Design review of the part built by this model. Coordinates are the model's own, in mm. Face numbers are marked on the shaded views. A direction names the side the tool comes from. Round coordinates to 2 decimals unless told otherwise and drop trailing zeros. Write each loop counter-clockwise with the first axis right and the second up, starting at its lowest first coordinate (ties: lowest second). Pieces come first, ordered by that corner, then holes. Notation, with made-up numbers: (-24, 33) - (-4, 33) arc R27 cw to (-4, 71) - close; hole circle Ø4 at (-13, 87.25). An arc over 180 degrees is marked (long way). Use one line per item in the form item = value.
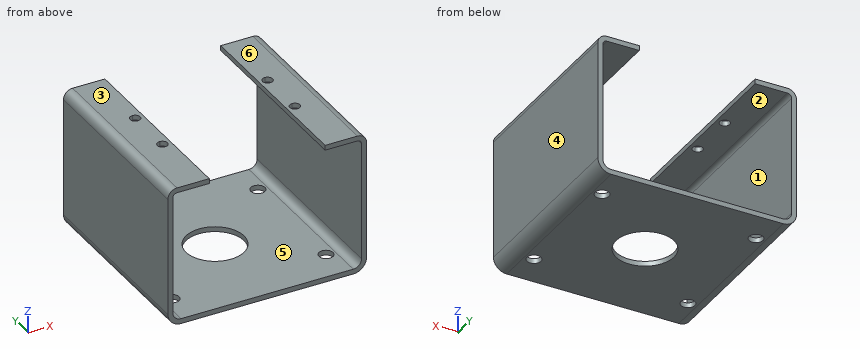
```python
from build123d import *

# Parameters (mm, degrees)
SKETCH1_W                      = 120
SKETCH1_H                      = 115
BASE_FLANGE1_DEPTH             = 3
EDGE_FLANGE1_STRIP_W           = 22
EDGE_FLANGE1_STRIP_H           = 3
EDGE_FLANGE1_STRIP_CUT_DEPTH   = 115
EDGE_FLANGE1_STRIP_2_W         = 22
EDGE_FLANGE1_STRIP_2_H         = 3
EDGE_FLANGE1_STRIP_CUT_2_DEPTH = 115
EDGE_FLANGE1_DEPTH             = 115
EDGE_FLANGE1_BEND_DEPTH        = 115
EDGE_FLANGE2_STRIP_W           = 17
EDGE_FLANGE2_STRIP_H           = 3
EDGE_FLANGE2_STRIP_CUT_DEPTH   = 115
EDGE_FLANGE2_STRIP_2_W         = 17
EDGE_FLANGE2_STRIP_2_H         = 3
EDGE_FLANGE2_STRIP_CUT_2_DEPTH = 115
EDGE_FLANGE2_DEPTH             = 115
EDGE_FLANGE2_BEND_DEPTH        = 115
CUT_EXTRUDE1_DEPTH             = 10
LPATTERN1_COUNT                = 2
LPATTERN1_PITCH                = 30
LPATTERN2_COUNT                = 2
LPATTERN2_PITCH                = 80
LPATTERN2_COPY_1_DEPTH         = 10
SKETCH19_R                     = 4.25
CUT_EXTRUDE2_DEPTH             = 10
LPATTERN3_COUNT                = 2
LPATTERN3_PITCH                = 75
SKETCH20_R                     = 17.5
CUT_EXTRUDE3_DEPTH             = 10


# Sheet-metal steps are written as plain solids
with BuildPart() as part:
    # Sketch1 → Base-Flange1 (new body)
    with BuildSketch(Plane.XY):
        Rectangle(SKETCH1_W, SKETCH1_H)
    extrude(amount=-BASE_FLANGE1_DEPTH)

    # Edge-Flange1 strip (across the edge) → Edge-Flange1 strip cut (cut)
    with BuildSketch(Plane(origin=(60, -57.5, 0), x_dir=(-1, 0, 0), z_dir=(0, 1, 0))):
        with Locations((-3, -1.5)):
            Rectangle(EDGE_FLANGE1_STRIP_W, EDGE_FLANGE1_STRIP_H)
    extrude(amount=EDGE_FLANGE1_STRIP_CUT_DEPTH, mode=Mode.SUBTRACT)

    # Edge-Flange1 strip 2 (across the edge) → Edge-Flange1 strip cut 2 (cut)
    with BuildSketch(Plane(origin=(-60, 57.5, 0), x_dir=(1, 0, 0), z_dir=(0, -1, 0))):
        with Locations((-3, -1.5)):
            Rectangle(EDGE_FLANGE1_STRIP_2_W, EDGE_FLANGE1_STRIP_2_H)
    extrude(amount=EDGE_FLANGE1_STRIP_CUT_2_DEPTH, mode=Mode.SUBTRACT)

    # Edge-Flange1 section (across the edge) → Edge-Flange1 (add)
    with BuildSketch(Plane(origin=(60, -57.5, 0), x_dir=(-1, 0, 0), z_dir=(0, 1, 0))):
        with BuildLine():
            Line((0, 5), (0, 82))
            Line((0, 82), (3, 82))
            Line((3, 82), (3, 5))
            ThreePointArc((3, 5), (4.464466094, 1.464466094), (8, 0))
            Line((8, 0), (8, -3))
            ThreePointArc((8, -3), (2.343145751, -0.656854249), (0, 5))
        make_face()
    extrude(amount=EDGE_FLANGE1_DEPTH)

    # Edge-Flange1 section 2 (across the edge) → Edge-Flange1 bend (add)
    with BuildSketch(Plane(origin=(-60, 57.5, 0), x_dir=(1, 0, 0), z_dir=(0, -1, 0))):
        with BuildLine():
            Line((0, 5), (0, 82))
            Line((0, 82), (3, 82))
            Line((3, 82), (3, 5))
            ThreePointArc((3, 5), (4.464466094, 1.464466094), (8, 0))
            Line((8, 0), (8, -3))
            ThreePointArc((8, -3), (2.343145751, -0.656854249), (0, 5))
        make_face()
    extrude(amount=EDGE_FLANGE1_BEND_DEPTH)

    # Edge-Flange2 strip (across the edge) → Edge-Flange2 strip cut (cut)
    with BuildSketch(Plane(origin=(-57, 57.5, 82), x_dir=(0, 0, -1), z_dir=(0, -1, 0))):
        with Locations((-3, -1.5)):
            Rectangle(EDGE_FLANGE2_STRIP_W, EDGE_FLANGE2_STRIP_H)
    extrude(amount=EDGE_FLANGE2_STRIP_CUT_DEPTH, mode=Mode.SUBTRACT)

    # Edge-Flange2 strip 2 (across the edge) → Edge-Flange2 strip cut 2 (cut)
    with BuildSketch(Plane(origin=(57, -57.5, 82), x_dir=(0, 0, -1), z_dir=(0, 1, 0))):
        with Locations((-3, -1.5)):
            Rectangle(EDGE_FLANGE2_STRIP_2_W, EDGE_FLANGE2_STRIP_2_H)
    extrude(amount=EDGE_FLANGE2_STRIP_CUT_2_DEPTH, mode=Mode.SUBTRACT)

    # Edge-Flange2 section (across the edge) → Edge-Flange2 (add)
    with BuildSketch(Plane(origin=(-57, 57.5, 82), x_dir=(0, 0, -1), z_dir=(0, -1, 0))):
        with BuildLine():
            Line((0, 2.5), (0, 22))
            Line((0, 22), (3, 22))
            Line((3, 22), (3, 2.5))
            ThreePointArc((3, 2.5), (3.732233047, 0.732233047), (5.5, 0))
            Line((5.5, 0), (5.5, -3))
            ThreePointArc((5.5, -3), (1.610912703, -1.389087297), (0, 2.5))
        make_face()
    extrude(amount=EDGE_FLANGE2_DEPTH)

    # Edge-Flange2 section 2 (across the edge) → Edge-Flange2 bend (add)
    with BuildSketch(Plane(origin=(57, -57.5, 82), x_dir=(0, 0, -1), z_dir=(0, 1, 0))):
        with BuildLine():
            Line((0, 2.5), (0, 22))
            Line((0, 22), (3, 22))
            Line((3, 22), (3, 2.5))
            ThreePointArc((3, 2.5), (3.732233047, 0.732233047), (5.5, 0))
            Line((5.5, 0), (5.5, -3))
            ThreePointArc((5.5, -3), (1.610912703, -1.389087297), (0, 2.5))
        make_face()
    extrude(amount=EDGE_FLANGE2_BEND_DEPTH)

    # Sketch18 → Cut-Extrude1 (cut)
    with BuildSketch(Plane.XY.offset(82)):
        with BuildLine():
            Line((-40.05, -12), (-39.95, -12))
            ThreePointArc((-39.95, -12), (-36.95, -15), (-39.95, -18))
            Line((-39.95, -18), (-40.05, -18))
            ThreePointArc((-40.05, -18), (-43.05, -15), (-40.05, -12))
        make_face()
    cut_extrude1 = extrude(amount=-CUT_EXTRUDE1_DEPTH, mode=Mode.SUBTRACT)

    # LPattern1: Cut-Extrude1 ×2
    with Locations(*[(0, i * LPATTERN1_PITCH, 0) for i in range(1, LPATTERN1_COUNT)]):
        add(cut_extrude1, mode=Mode.SUBTRACT)

    # LPattern2: Cut-Extrude1 ×2
    with Locations(*[(i * LPATTERN2_PITCH, 0, 0) for i in range(1, LPATTERN2_COUNT)]):
        add(cut_extrude1, mode=Mode.SUBTRACT)

    # LPattern2 copy 1 sketch → LPattern2 copy 1 (cut)
    with BuildSketch(Plane(origin=(80, 30, 82), x_dir=(1, 0, 0), z_dir=(0, 0, 1))):
        with BuildLine():
            Line((-40.05, -12), (-39.95, -12))
            ThreePointArc((-39.95, -12), (-36.95, -15), (-39.95, -18))
            Line((-39.95, -18), (-40.05, -18))
            ThreePointArc((-40.05, -18), (-43.05, -15), (-40.05, -12))
        make_face()
    extrude(amount=-LPATTERN2_COPY_1_DEPTH, mode=Mode.SUBTRACT)

    # Sketch19 → Cut-Extrude2 (cut)
    with BuildSketch(Plane(origin=(0, 0, -3), x_dir=(-1, 0, 0), z_dir=(0, 0, -1))):
        with Locations((-46.5, -37.5)):
            Circle(SKETCH19_R)
        with Locations((46.5, -37.5)):
            Circle(SKETCH19_R)
    cut_extrude2 = extrude(amount=-CUT_EXTRUDE2_DEPTH, mode=Mode.SUBTRACT)

    # LPattern3: Cut-Extrude2 ×2
    with Locations(*[(0, i * LPATTERN3_PITCH, 0) for i in range(1, LPATTERN3_COUNT)]):
        add(cut_extrude2, mode=Mode.SUBTRACT)

    # Sketch20 → Cut-Extrude3 (cut)
    with BuildSketch(Plane(origin=(0, 0, -3), x_dir=(-1, 0, 0), z_dir=(0, 0, -1))):
        Circle(SKETCH20_R)
    extrude(amount=-CUT_EXTRUDE3_DEPTH, mode=Mode.SUBTRACT)


solid = part.part
```
Q1. For P1, Ø0.9, axis at y = -5.5, z = 80, coming from the +X side; P2, Ø6, axis at x = 14.5, y = 5.5, coming from the +Z side; P3, Ø1.5, axis at y = -22.5, z = 80.5, coming from the -X side, all flat-tipped, find the tip position at first contact; note any pin that passes through.
Calculated:
P1 = 59.08
P2 = 0
P3 = -58.94
Q2. We need section B-B on z = 15. Write out the cut boundary in (x, y), then the cut area to 3 significant figures.
Calculated:
outline = (-60, -57.5) - (-57, -57.5) - (-57, 57.5) - (-60, 57.5) - close; (57, -57.5) - (60, -57.5) - (60, 57.5) - (57, 57.5) - close
area = 690 mm2
Q3. We need section D-D on x = -9.5. Write out the cut boundary in (y, z), then the cut area to 3 significant figures.
Calculated:
outline = (-57.5, -3) - (-14.7, -3) - (-14.7, 0) - (-57.5, 0) - close; (14.7, -3) - (57.5, -3) - (57.5, 0) - (14.7, 0) - close
area = 257 mm2
Q4. We need section C-C on y = 15. State how many separate pieces and enclosed holes the cut face has, then the cut area to 3 significant figures.
Calculated:
separate_pieces = 4
enclosed_holes = 0
area = 866 mm2
Q5. Machinability: for the marked faces 5 and 6, which of the approach directions +Z, -Z, +X, -X, +Y, -Y give a long, thin tool a straight path to every point of the face, cutting with its end or side? Answer none if there is none.
Calculated:
face_5 = +Y, -Y
face_6 = +Z, +X, -X, +Y, -Y
Q6. To check wall thickness, follow line 1 along X through (y, z) = (39, 36); line 2 along Y through (x, z) = (-46.5, -1.3); line 3 along Z through (x, y) = (-38, -19.5). State the ranges of each line that lie inside material, in increasing order. Write a range as from..to.
Calculated:
line_1 = -60..-57, 57..60
line_2 = -57.5..-41.75, -33.25..33.25, 41.75..57.5
line_3 = -3..0, 79..82
Q7. We need section A-A on y = 37.5. Write out the cut boundary in (x, z), then the cut area to 3 significant figures.
Calculated:
outline = (-60, 5) arc R8 ccw to (-52, -3) - (-50.75, -3) - (-50.75, 0) - (-52, 0) arc R5 cw to (-57, 5) - (-57, 76.5) arc R2.5 cw to (-54.5, 79) - (-35, 79) - (-35, 82) - (-54.5, 82) arc R5.5 ccw to (-60, 76.5) - close; (-42.25, -3) - (42.25, -3) - (42.25, 0) - (-42.25, 0) - close; (35, 79) - (54.5, 79) arc R2.5 cw to (57, 76.5) - (57, 5) arc R5 cw to (52, 0) - (50.75, 0) - (50.75, -3) - (52, -3) arc R8 ccw to (60, 5) - (60, 76.5) arc R5.5 ccw to (54.5, 82) - (35, 82) - close
area = 906 mm2
Q8. Draft analysis for pull direction X (two halves, no side actions). For the marked faces 1, 2, 3 and 4, state which applies: released by +X, released by -X, zero draft, split by the parting line, or undercut.
Calculated:
face_1 = undercut
face_2 = undercut
face_3 = zero draft
face_4 = released by +X
